For this review, take the finished solid that the model builds, in its own axes (mm). Face numbers are marked on the shaded views. A direction names the side the tool comes from. Coordinates: 2 decimals unless noted, no trailing zeros. Loops run counter-clockwise (first coordinate to the right, second up) from the corner with the lowest first, then second, coordinate; pieces in that order, holes last. Notation, with made-up numbers: (19, -14) - (52, -14) arc R20 cw to (52, -2) - close; hole circle Ø11 at (1, 58). An arc over 180 degrees is marked (long way). Answer as a JSON object with one key per item and string values. Group by question number.
Item 1: To check wall thickness, follow line 1 (Y direction, x = 20, z = 29) (3 decimals); line 2 (Y direction, x = 18, z = 29); line 3 (Z direction, x = 6, y = 1.5). State the ranges of each line that lie inside material, in increasing order.
Item 2: We need section B-B (x = 20). Give the boundary of the cut face in (y, z) (3 decimals).
Item 3: We need section D-D (x = 38.5). Give the boundary of the cut face in (y, z), then the cut area to 3 significant figures.
Item 4: Tool access review of the marked faces 1 and 2: name each direction out of +Z, -Z, +X, -X, +Y, -Y from which nothing blocks a thin tool from reaching the whole face with its end or side.
Item 5: Clearance check with flat-ended pins moving along their axes: pin 1 (1 mm diameter, centred on y = 6.5, z = 12.5, fed in from +X); pin 2 (4 mm diameter, centred on y = 2, z = 20.5, fed in from -X); pin 3 (2 mm diameter, centred on x = 7.5, y = 5.5, fed in from +Z). State where each tip first meets the part, or that it passes through.
Item 6: We need section A-A (y = 7). Give the boundary of the cut face in (x, z) (3 decimals), then the cut area to 3 significant figures.
Item 7: We need section C-C (z = 15). Give the boundary of the cut face in (x, y).
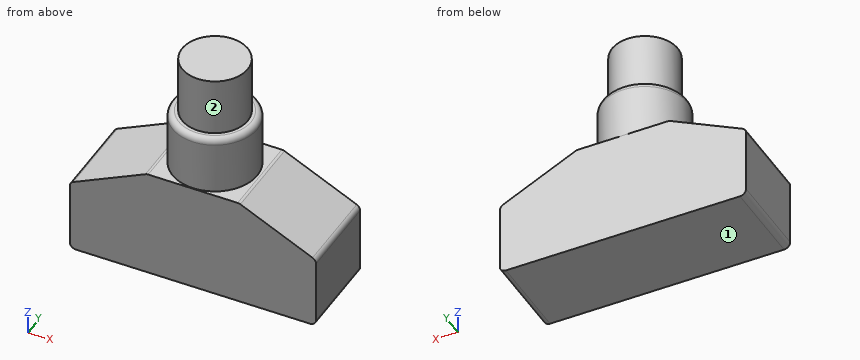
from build123d import *

# Parameters (mm, degrees)
BOSS_EXTRUDE1_DEPTH = 14
SKETCH2_R           = 6.875
BOSS_EXTRUDE2_DEPTH = 9.5
SKETCH3_R           = 5.325
BOSS_EXTRUDE3_DEPTH = 9.5
FILLET1_R           = 1


with BuildPart() as part:
    # Sketch1 → Boss-Extrude1 (new body)
    with BuildSketch(Plane(origin=(0, 0, 0), x_dir=(1, 0, 0), z_dir=(0, 1, 0))):
        Polygon((0, 0), (0, -12), (12.5, -18), (27.5, -18), (40, -12), (40, 0), align=None)
    extrude(amount=BOSS_EXTRUDE1_DEPTH)

    # Sketch2 → Boss-Extrude2 (add)
    with BuildSketch(Plane.XY.offset(18)):
        with Locations((20, 7)):
            Circle(SKETCH2_R)
    extrude(amount=BOSS_EXTRUDE2_DEPTH)

    # Sketch3 → Boss-Extrude3 (add)
    with BuildSketch(Plane.XY.offset(27.5)):
        with Locations((20, 7)):
            Circle(SKETCH3_R)
    extrude(amount=BOSS_EXTRUDE3_DEPTH)

    # Fillet1
    fillet1_edges = [part.edges().sort_by_distance(p)[0] for p in [
        (0, 7, 0),
        (40, 7, 0),
        (40, 7, 12),
        (27.5, 7, 18),
        (12.5, 7, 18),
        (0, 7, 12),
        (13.125, 7, 27.5),
    ]]
    fillet(fillet1_edges, radius=FILLET1_R)


solid = part.part
Check sheet entries:
{
 "1": {"line 1": "y = 1.675 to 12.325", "line 2": "y = 2.06 to 11.94", "line 3": "z = 0 to 14.88"},
 "2": {"outline": "(0, 0) - (14, 0) - (14, 18) - (13.875, 18) - (13.875, 26.5) arc R1 ccw to (12.875, 27.5) - (12.325, 27.5) - (12.325, 37) - (1.675, 37) - (1.675, 27.5) - (1.125, 27.5) arc R1 ccw to (0.125, 26.5) - (0.125, 18) - (0, 18) - close"},
 "3": {"outline": "(0, 0) - (14, 0) - (14, 12.72) - (0, 12.72) - close", "area": "178 mm2"},
 "4": {"face 1": "-Z, +X, -X, +Y, -Y", "face 2": "+Z"},
 "5": {"pin 1": "stops at x = 39.78", "pin 2": "stops at x = 13.81", "pin 3": "stops at z = 16.08"},
 "6": {"outline": "(0, 1) arc R1 ccw to (1, 0) - (39, 0) arc R1 ccw to (40, 1) - (40, 11.371) arc R1 ccw to (39.433, 12.272) - (27.705, 17.902) arc R1 ccw to (27.272, 18) - (26.875, 18) - (26.875, 26.5) arc R1 ccw to (25.875, 27.5) - (25.325, 27.5) - (25.325, 37) - (14.675, 37) - (14.675, 27.5) - (14.125, 27.5) arc R1 ccw to (13.125, 26.5) - (13.125, 18) - (12.728, 18) arc R1 ccw to (12.295, 17.902) - (0.567, 12.272) arc R1 ccw to (0, 11.371) - close", "area": "876 mm2"},
 "7": {"outline": "(6.25, 0) - (33.75, 0) - (33.75, 14) - (6.25, 14) - close"}
}
